Could you check a few things on this model? Use its own coordinates, in mm. Face numbers are marked on the shaded views. A direction names the side the tool comes from. Give positions to 0.01 mm unless a question says otherwise; leave off trailing zeros. Loops run counter-clockwise (first coordinate to the right, second up) from the corner with the lowest first, then second, coordinate; pieces in that order, holes last. Notation, with made-up numbers: M -18.5,-24.75 L 14.5,-24.75 A15 cw 14.5,0.25 Z; hole C 73.5,36.25 d8. An arc over 180 degrees is marked long. Answer in a Markdown table with one row per item. Add a question column.
1. If we section it at B-B on x = 0: List the corners of the cut face in (y, z) for me (3 decimals).
2. Which directions (+Z, -Z, +X, -X, +Y, -Y) give clear straight access to the entire face, cutting with the end or side of a thin tool? Please do the marked faces 5 and 6.
3. Thinking about a two-plate mould opening in Y: for the marked faces 1, 2, 3 and 4, which applies, released by +Y, released by -Y, zero draft, split by the parting line, or undercut?
4. If we section it at A-A on z = 29: List the corners of the cut face in (x, y) for me, then the cut area to 3 significant figures.
5. I need wall thicknesses on line 1 along Y through (x, z) = (-30, 8.5); line 2 along Y through (x, z) = (-44, -27); line 3 along Z through (x, y) = (16, -138). Which ranges of each line are inside material? Lowest first, please. Write a range as from..to.
6. I'm going to push flat-ended pins straight in: pin 1 Ø3 at (x, z) = (31.5, -22.5) entering from +Y; pin 2 Ø4 at (x, z) = (34.5, 0) entering from +Y; pin 3 Ø8 at (x, z) = (-2.5, -17) entering from +Y; pin 4 Ø10 at (x, y) = (-4, -80.5) entering from +Z. Where does each tip first touch, or does it pass through?
7. If we section it at C-C on z = 0: List the corners of the cut face in (x, y) for me (3 decimals), then the cut area to 3 significant figures.
8. If we section it at D-D on y = -147.5: List the corners of the cut face in (x, z) for me.
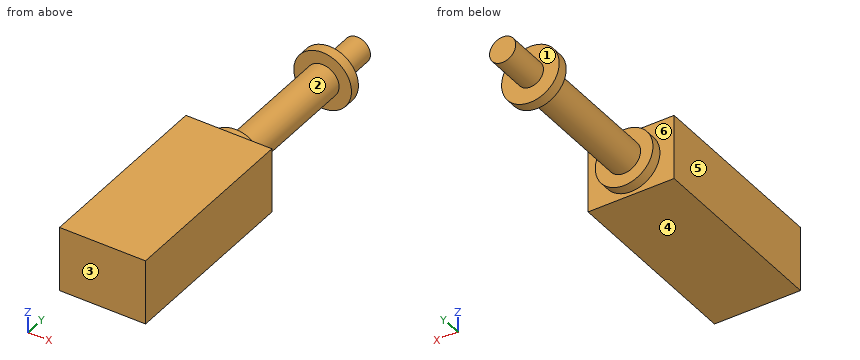
```python
from build123d import *

# Parameters (mm, degrees)
SKETCH1_R      = 34.925
EXTRUDE1_DEPTH = 12.7
SKETCH2_R      = 19.86600399
EXTRUDE2_DEPTH = 184.15
SKETCH3_R      = 15.875
EXTRUDE3_DEPTH = 50.8
EXTRUDE4_START = -12.7
SKETCH4_R      = 34.925
EXTRUDE4_DEPTH = 12.7
SKETCH5_W      = 104.14
SKETCH5_H      = 78.74
EXTRUDE5_DEPTH = 231.14


with BuildPart() as part:
    # Sketch1 → Extrude1 (new body)
    with BuildSketch(Plane(origin=(0, 0, 0), x_dir=(1, 0, 0), z_dir=(0, 1, 0))):
        with Locations(Location((0, 0, 0), (0, 0, 270))):
            Circle(SKETCH1_R)
    extrude(amount=-EXTRUDE1_DEPTH)

    # Sketch2 → Extrude2 (add)
    with BuildSketch(Plane(origin=(0, 0, 0), x_dir=(1, 0, 0), z_dir=(0, 1, 0))):
        with Locations(Location((0, 0, 0), (0, 0, 270))):
            Circle(SKETCH2_R)
    extrude(amount=-EXTRUDE2_DEPTH)

    # Sketch3 → Extrude3 (add)
    with BuildSketch(Plane(origin=(0, 0, 0), x_dir=(1, 0, 0), z_dir=(0, 1, 0))):
        with Locations(Location((0, 0, 0), (0, 0, 270))):
            Circle(SKETCH3_R)
    extrude(amount=EXTRUDE3_DEPTH)

    # Sketch4 → Extrude4 (add)
    with BuildSketch(Plane.XZ.offset(184.15).offset(EXTRUDE4_START)):
        with Locations(Location((0, 0, 0), (0, 0, 90))):
            Circle(SKETCH4_R)
    extrude(amount=EXTRUDE4_DEPTH)

    # Sketch5 → Extrude5 (add)
    with BuildSketch(Plane.XZ.offset(184.15)):
        Rectangle(SKETCH5_W, SKETCH5_H)
    extrude(amount=EXTRUDE5_DEPTH)


solid = part.part
```
Results:
| question | item | result |
|---|---|---|
| 1 | outline | M -415.29,-39.37 L -184.15,-39.37 L -184.15,-34.925 L -171.45,-34.925 L -171.45,-19.866 L -12.7,-19.866 L -12.7,-34.925 L 0,-34.925 L 0,-15.875 L 50.8,-15.875 L 50.8,15.875 L 0,15.875 L 0,34.925 L -12.7,34.925 L -12.7,19.866 L -171.45,19.866 L -171.45,34.925 L -184.15,34.925 L -184.15,39.37 L -415.29,39.37 Z |
| 2 | face 5 | +Z, -Z, -X, +Y, -Y |
| 2 | face 6 | +Y |
| 3 | face 1 | released by +Y |
| 3 | face 2 | undercut |
| 3 | face 3 | released by -Y |
| 3 | face 4 | zero draft |
| 4 | outline | M -52.07,-415.29 L 52.07,-415.29 L 52.07,-184.15 L 19.46,-184.15 L 19.46,-171.45 L -19.46,-171.45 L -19.46,-184.15 L -52.07,-184.15 Z; M -19.46,-12.7 L 19.46,-12.7 L 19.46,0 L -19.46,0 Z |
| 4 | area | 25,100 mm2 |
| 5 | line 1 | -415.29..-171.45, -12.7..0 |
| 5 | line 2 | -415.29..-184.15 |
| 5 | line 3 | -11.78..11.78 |
| 6 | pin 1 | y = -184.15 |
| 6 | pin 2 | y = 0 |
| 6 | pin 3 | y = 50.8 |
| 6 | pin 4 | z = 19.87 |
| 7 | outline | M -52.07,-415.29 L 52.07,-415.29 L 52.07,-184.15 L 34.925,-184.15 L 34.925,-171.45 L 19.866,-171.45 L 19.866,-12.7 L 34.925,-12.7 L 34.925,0 L 15.875,0 L 15.875,50.8 L -15.875,50.8 L -15.875,0 L -34.925,0 L -34.925,-12.7 L -19.866,-12.7 L -19.866,-171.45 L -34.925,-171.45 L -34.925,-184.15 L -52.07,-184.15 Z |
| 7 | area | 33,800 mm2 |
| 8 | outline | C 0,0 d39.73 |
